```python
from build123d import *

# Parameters (mm, degrees)
F1_DEPTH = 2.54
F2_R     = 2.6712032827
F3_DEPTH = 2.54


# Not quite as in the source:
# - the program builds the solid bodies; features that only make, move or delete a surface that nothing else refers to are left out


with BuildPart() as f1:
    # F0 (on Front) → F1 (new body)
    with BuildSketch(Plane.XZ):
        Polygon((-38.4220704436, 27.1976441145), (-38.9976799488, 23.4561692923), (-20.0024992228, 23.4561692923), (-20.0024992228, 35.8318164945), (-24.3195872754, 35.8318164945), (-24.3195872754, 31.2269236892), (-24.3195872754, 27.1976441145), align=None)
    extrude(amount=F1_DEPTH)

    # F2 (on Right) → F3 (cut)
    with BuildSketch(Plane.YZ):
        with Locations((0, 48.1319762766)):
            Circle(F2_R)
    extrude(amount=-F3_DEPTH, mode=Mode.SUBTRACT)


solid = f1.part
```
Here's how the part is built. I have some questions about the finished solid (model axes, mm). A direction names the side the tool comes from. Give positions to 0.01 mm unless a question says otherwise; leave off trailing zeros. Write each loop counter-clockwise with the first axis right and the second up, starting at its lowest first coordinate (ties: lowest second). Pieces come first, ordered by that corner, then holes. Notation, with made-up numbers: (25.5, 80) -> (43.5, 80) arc R7 cw to (43.5, 89) -> close; hole circle Ø8 at (-28, 13.5). An arc over 180 degrees is marked (long way). Write each question's results on one line, items separated by ' | '.
Item 1: On a 3-axis mill with a long thin cutter (end or side, diameter ignored), from which of +Z, -Z, +X, -X, +Y, -Y can I reach the whole of each face in a straight line? I mean faces 1 (the face through (-28, -2.54, 27)), 2 (the face through (-24.32, -1, 32)). Say none if no direction works.
Output:
face 1: +Z, -Z, +X, -X, -Y | face 2: +Z, -X, +Y, -Y
Item 2: Suppose I cut it at C-C on x = -36.5. Write out the boundary of the cut face in (y, z).
Output:
outline: (-2.54, 23.46) -> (0, 23.46) -> (0, 27.2) -> (-2.54, 27.2) -> close
Item 3: If I drill on L1, parallel to X at y = -0.9, z = 29.5; L2, parallel to Z at x = -25.25, y = -1.6; L3, parallel to X at y = -0.55, z = 24.25, over which ranges is the centre line in solid material (lowest first)?
Output:
L1: x = -24.32 to -20 | L2: z = 23.46 to 27.2 | L3: x = -38.88 to -20
Item 4: Suppose I cut it at A-A on y = -1.75. Write out the boundary of the cut face in (x, z).
Output:
outline: (-39, 23.46) -> (-20, 23.46) -> (-20, 35.83) -> (-24.32, 35.83) -> (-24.32, 27.2) -> (-38.42, 27.2) -> close
Item 5: For pin 1 Ø1.5 at (x, z) = (-28.5, 29) entering from -Y, with a flat end and sliding along its axis, tell me the tip position at first contact or that it passes through.
Output:
pin 1: passes through
Item 6: Suppose I cut it at B-B on z = 33.25. Write out the boundary of the cut face in (x, y), plus the area to 3 significant figures.
Output:
outline: (-24.32, -2.54) -> (-20, -2.54) -> (-20, 0) -> (-24.32, 0) -> close | area: 11.0 mm^2
